from build123d import *

# Parameters (mm, degrees)
CROQUIS1_R              = 4.5
CROQUIS1_R_2            = 1.249999997
CROQUIS1_R_3            = 1.25
CROQUIS1_R_4            = 1.250000007
CROQUIS1_R_5            = 1.55
SALIENTE_EXTRUIR1_DEPTH = 1.6


with BuildPart() as part:
    # Croquis1 → Saliente-Extruir1 (new body)
    with BuildSketch(Plane.XY):
        with BuildLine():
            Line((-18.876999997, -10.553790007), (18.892053472, -10.553790007))
            Line((18.892053472, -10.553790007), (18.892053472, -5.910945686))
            add(Edge.make_bspline(
                [(18.892053472, -5.910945686), (18.378347588, -0.392416566), (14.881416045, 2.073879198)],
                knots=[0, 0, 0, 0.734097382, 0.734097382, 0.734097382], degree=2))
            Line((14.881416045, 2.073879198), (9.601527182, 8.142540641))
            ThreePointArc((9.601527182, 8.142540641), (-0.182204471, 12.944844806), (-9.816792732, 7.849407753))
            Line((-9.816792732, 7.849407753), (-14.886628426, 2.036126845))
            add(Edge.make_bspline(
                [(-18.876999997, -5.958845057), (-18.377293132, -0.43903071), (-14.886628426, 2.036126845)],
                knots=[0, 0, 0, 0.734097382, 0.734097382, 0.734097382], degree=2))
            Line((-18.876999997, -5.958845057), (-18.876999997, -10.553790007))
        make_face()
        with Locations((-0.0012, 0.946209993)):
            Circle(CROQUIS1_R, mode=Mode.SUBTRACT)
        with Locations((-0.0024, 6.945010003)):
            Circle(CROQUIS1_R_2, mode=Mode.SUBTRACT)
        with Locations((5.193313192, 3.946649223)):
            Circle(CROQUIS1_R_3, mode=Mode.SUBTRACT)
        with Locations((5.194513192, -2.052150777)):
            Circle(CROQUIS1_R_3, mode=Mode.SUBTRACT)
        with Locations((0, -5.052590007)):
            Circle(CROQUIS1_R_3, mode=Mode.SUBTRACT)
        with Locations((-5.195713192, -2.054229238)):
            Circle(CROQUIS1_R_3, mode=Mode.SUBTRACT)
        with Locations((-5.196913248, 3.944570795)):
            Circle(CROQUIS1_R_4, mode=Mode.SUBTRACT)
        with Locations((12.6988, -3.853790007)):
            Circle(CROQUIS1_R_5, mode=Mode.SUBTRACT)
        with Locations((-12.6988, -3.853790007)):
            Circle(CROQUIS1_R_5, mode=Mode.SUBTRACT)
    extrude(amount=SALIENTE_EXTRUIR1_DEPTH)


solid = part.part
Part model, mm, in its own coordinate system. Round coordinates to 2 decimals unless told otherwise and drop trailing zeros. Order: outer loops, then holes, each group sorted by start corner. A loop starts at its lowest first (then second) coordinate and runs counter-clockwise, first axis right, second up. Notation, with made-up numbers: (51, 32.25) -> (89, 32.25) arc R17 cw to (89, 46.25) -> close; hole circle Ø10 at (11.5, -16.5). An arc over 180 degrees is marked (long way). Put each result on its own line as item: value.
Q1. Band-saw the part on A-A (x = -5.5). Give the cut face in (y, z).
From the geometry:
outline: (-10.55, 0) -> (-3.27, 0) -> (-3.27, 1.6) -> (-10.55, 1.6) -> close; (-0.84, 0) -> (2.73, 0) -> (2.73, 1.6) -> (-0.84, 1.6) -> close; (5.16, 0) -> (11.61, 0) -> (11.61, 1.6) -> (5.16, 1.6) -> close
Q2. Pull direction Y, two halves, no side cores. Call faces 1 (the face through (4, -4, 1.6)), 2 (the face through (-4.003, -1.679, 0.789)), 3 (the face through (-12.3, 5, 0.8)), 4 (the face through (6.386, 4.322, 0.789)): pulls with the +Y half, pulls with the -Y half, needs draft (parallel to the pull), parting line crosses it, or undercut.
From the geometry:
face 1: needs draft
face 2: undercut
face 3: pulls with the +Y half
face 4: undercut
Q3. Band-saw the part on C-C (z = 0.4). State how many separate pieces and enclosed holes the cut face has, and give its area (3 significant figures).
From the geometry:
separate pieces: 1
enclosed holes: 9
area: 562 mm2
Q4. Wall check: line 1 (Y direction, x = 0, z = 0.45) (3 decimals); line 2 (X direction, y = -3, z = 1.35); line 3 (X direction, y = 4.5, z = 0.95). Give the ranges that are in metal, low to high. Write a range as [from, to].
From the geometry:
line 1: y = [-10.554, -6.303], [-3.803, -3.554], [5.446, 5.695], [8.195, 12.946]
line 2: x = [-18.33, -13.99], [-11.41, -6.01], [-4.38, -2.16], [2.16, 4.38], [6.01, 11.41], [13.99, 18.35]
line 3: x = [-12.74, -6.32], [-4.08, -2.76], [2.76, 4.07], [6.31, 12.77]
Q5. Band-saw the part on D-D (x = -10.5). Give the cut face in (y, z), and give its area (3 significant figures).
From the geometry:
outline: (-10.55, 0) -> (7.07, 0) -> (7.07, 1.6) -> (-10.55, 1.6) -> close
area: 28.2 mm2
Q6. Pin check, flat tip, straight feed: pin 1 Ø1.5 at (x, y) = (-5.2, -2.05) entering from +Z. Stop position of the tip, or through.
From the geometry:
pin 1: passes through
Q7. Band-saw the part on B-B (x = 0). Give the cut face in (y, z) (3 decimals), and give its area (3 significant figures).
From the geometry:
outline: (-10.554, 0) -> (-6.303, 0) -> (-6.303, 1.6) -> (-10.554, 1.6) -> close; (-3.803, 0) -> (-3.554, 0) -> (-3.554, 1.6) -> (-3.803, 1.6) -> close; (5.446, 0) -> (5.695, 0) -> (5.695, 1.6) -> (5.446, 1.6) -> close; (8.195, 0) -> (12.946, 0) -> (12.946, 1.6) -> (8.195, 1.6) -> close
area: 15.2 mm2
